```python
from build123d import *

# Parameters (mm, degrees)
SKETCH1_W               = 90
SKETCH1_H               = 52
BOSS_EXTRUDE1_DEPTH     = 3
BOSS_EXTRUDE2_START     = 3
SKETCH4_R               = 2.5
BOSS_EXTRUDE2_DEPTH     = 7
CUT_EXTRUDE2_DEPTH      = 53.92447449
CUT_EXTRUDE2_DEPTH_BACK = 63.92447449
CUT_EXTRUDE2_START      = 10
SKETCH5_R               = 1.35
BOSS_EXTRUDE3_START     = 10
SKETCH6_R               = 0.9
BOSS_EXTRUDE3_DEPTH     = 12.5
SKETCH7_W               = 87
SKETCH7_H               = 49
SKETCH7_W_2             = 81
SKETCH7_H_2             = 43
BOSS_EXTRUDE4_DEPTH     = 2
FILLET1_R               = 3
BOSS_EXTRUDE8_START     = 3
SKETCH8_W               = 89
SKETCH8_H               = 51
SKETCH8_W_2             = 84
SKETCH8_H_2             = 46
BOSS_EXTRUDE8_DEPTH     = 20
FILLET2_R               = 2
CUT_EXTRUDE3_START      = 42
SKETCH9_W               = 14
SKETCH9_H               = 7
CUT_EXTRUDE3_DEPTH      = 15
BOSS_EXTRUDE9_START     = 44.5
BOSS_EXTRUDE9_DEPTH     = 0.2


with BuildPart() as part:
    # Sketch1 → Boss-Extrude1 (new body)
    with BuildSketch(Plane(origin=(0, 0, 0), x_dir=(1, 0, 0), z_dir=(0, 1, 0))):
        Rectangle(SKETCH1_W, SKETCH1_H)
    extrude(amount=BOSS_EXTRUDE1_DEPTH)

    # Sketch4 → Boss-Extrude2 (add)
    with BuildSketch(Plane(origin=(0, 0, 0), x_dir=(1, 0, 0), z_dir=(0, 1, 0)).offset(BOSS_EXTRUDE2_START)):
        with Locations(Location((29, -19.5, 0), (0, 0, 270))):
            Circle(SKETCH4_R)
        with Locations(Location((-37, 18, 0), (0, 0, 270))):
            Circle(SKETCH4_R)
        with Locations(Location((-37, -16.5, 0), (0, 0, 270))):
            Circle(SKETCH4_R)
    extrude(amount=BOSS_EXTRUDE2_DEPTH)

    # Sketch5 → Cut-Extrude2 (cut, two sides: drawn at the far end of the back side and taken through both)
    with BuildSketch(Plane(origin=(0, 0, 0), x_dir=(1, 0, 0), z_dir=(0, 1, 0)).offset(CUT_EXTRUDE2_START - CUT_EXTRUDE2_DEPTH_BACK)):
        with Locations(Location((-37, 18, 0), (0, 0, 270))):
            Circle(SKETCH5_R)
        with Locations(Location((-37, -16.5, 0), (0, 0, 270))):
            Circle(SKETCH5_R)
    extrude(amount=CUT_EXTRUDE2_DEPTH + CUT_EXTRUDE2_DEPTH_BACK, mode=Mode.SUBTRACT)

    # Sketch6 → Boss-Extrude3 (add)
    with BuildSketch(Plane(origin=(0, 0, 0), x_dir=(1, 0, 0), z_dir=(0, 1, 0)).offset(BOSS_EXTRUDE3_START)):
        with Locations(Location((29, -19.5, 0), (0, 0, 270))):
            Circle(SKETCH6_R)
    extrude(amount=BOSS_EXTRUDE3_DEPTH)

    # Sketch7 → Boss-Extrude4 (add)
    with BuildSketch(Plane(origin=(0, 0, 0), x_dir=(1, 0, 0), z_dir=(0, 1, 0))):
        Rectangle(SKETCH7_W, SKETCH7_H)
        Rectangle(SKETCH7_W_2, SKETCH7_H_2, mode=Mode.SUBTRACT)
    extrude(amount=-BOSS_EXTRUDE4_DEPTH)

    # Fillet1
    fillet1_edges = [part.edges().sort_by_distance(p)[0] for p in [
        (43.5, -1, -24.5),
        (43.5, -1, 24.5),
        (-43.5, -1, 24.5),
        (-43.5, -1, -24.5),
    ]]
    fillet(fillet1_edges, radius=FILLET1_R)

    # Sketch8 → Boss-Extrude8 (add)
    with BuildSketch(Plane(origin=(0, 0, 0), x_dir=(1, 0, 0), z_dir=(0, 1, 0)).offset(BOSS_EXTRUDE8_START)):
        Rectangle(SKETCH8_W, SKETCH8_H)
        Rectangle(SKETCH8_W_2, SKETCH8_H_2, mode=Mode.SUBTRACT)
    extrude(amount=BOSS_EXTRUDE8_DEPTH)

    # Fillet2
    fillet2_edges = [part.edges().sort_by_distance(p)[0] for p in [
        (44.5, 13, -25.5),
        (-44.5, 13, -25.5),
        (-44.5, 13, 25.5),
        (44.5, 13, 25.5),
        (-45, 1.5, -26),
        (45, 1.5, -26),
        (45, 1.5, 26),
        (-45, 1.5, 26),
    ]]
    fillet(fillet2_edges, radius=FILLET2_R)

    # Sketch9 → Cut-Extrude3 (cut)
    with BuildSketch(Plane(origin=(0, 0, 0), x_dir=(0, 0, -1), z_dir=(1, 0, 0)).offset(CUT_EXTRUDE3_START)):
        with Locations((11, 6.5)):
            Rectangle(SKETCH9_W, SKETCH9_H)
    extrude(amount=CUT_EXTRUDE3_DEPTH, mode=Mode.SUBTRACT)

    # Sketch10 → Boss-Extrude9 (add)
    with BuildSketch(Plane(origin=(0, 0, 0), x_dir=(0, 0, -1), z_dir=(1, 0, 0)).offset(BOSS_EXTRUDE9_START)):
        Polygon((18, 3), (18, 10), (4, 10), (4, 3), (3, 3), (3, 11), (19, 11), (19, 3), align=None)
    extrude(amount=BOSS_EXTRUDE9_DEPTH)


solid = part.part
```
Verification items for the finished model (mm, model axes). A direction names the side the tool comes from. Coordinates: 2 decimals unless noted, no trailing zeros. Order: outer loops, then holes, each group sorted by start corner. A loop starts at its lowest first (then second) coordinate and runs counter-clockwise, first axis right, second up. Notation, with made-up numbers: (49.25, 18.5) -> (76.25, 18.5) arc R13 ccw to (76.25, 33.5) -> close; hole circle Ø9 at (5, -2.5). An arc over 180 degrees is marked (long way). Answer as CSV lines item,"result". Start each with the question number.
1) Cross-section at A-A, the plane y = 16. Record the boundary of the cut face in (x, z), then the cut area to 3 significant figures.
2) Material ranges on L1, parallel to X at y = 5, z = 16.5; L2, parallel to Z at x = 4.5, y = 21.25; L3, parallel to X at y = 4.5, z = 9, recorded low to high. Write a range as [from, to].
3) Set-up check for faces 1 (the face through (44.7, 10.3, -11)), 2 (the face through (-38.1, 10, -16.9)), 3 (the face through (-43.9, 13.14, -24.93)): record each of +Z, -Z, +X, -X, +Y, -Y from which the full face is reachable in a straight line by a thin tool's end or side.
4) Cross-section at D-D, the plane x = -37. Give the number of separate pieces and of enclosed holes in the cut face, then the cut area to 3 significant figures.
5) Cross-section at C-C, the plane z = 5. Record the boundary of the cut face in (x, y).
6) Gauge pin test, flat ends, axial feed: pin 1 Ø1.6 at (x, y) = (-1, -1.5) entering from -Z; pin 2 Ø2 at (y, z) = (11, 1) entering from +X; pin 3 Ø4 at (x, y) = (-18, 10.5) entering from -Z. Record the tip position at first contact, or that the pin passes through.
7) Release check for a two-part mould opening along X. For faces 4 (the face through (43.93, 13.14, -24.9)), 5 (the face through (-38.32, 4.93, 16.21)), 6 (the face through (-1, -1, 24.5)) record: released by +X, released by -X, zero draft, split by the parting line, or undercut.
8) Cross-section at B-B, the plane x = 29. Record the boundary of the cut face in (y, z).
Conclusion:
1,outline,"(-44.5, -23.5) arc R2 ccw to (-42.5, -25.5) -> (42.5, -25.5) arc R2 ccw to (44.5, -23.5) -> (44.5, 23.5) arc R2 ccw to (42.5, 25.5) -> (-42.5, 25.5) arc R2 ccw to (-44.5, 23.5) -> close; circle Ø1.8 at (29, 19.5); hole (-42, -23) -> (42, -23) -> (42, 23) -> (-42, 23) -> close"
1,area,"674 mm²"
2,L1,"x = [-44.5, -42], [-39.5, -38.35], [-35.65, -34.5], [42, 44.5]"
2,L2,"z = [-25.5, -23], [23, 25.5]"
2,L3,"x = [-44.5, -42], [42, 44.5]"
3,face 1,"+Z, -Z, +X, +Y"
3,face 2,"+Y"
3,face 3,"-Z, -X, +Y"
4,separate pieces,"3"
4,enclosed holes,"0"
4,area,"284 mm²"
5,outline,"(-45, 0) -> (-43.5, 0) -> (-43.5, -2) -> (-40.5, -2) -> (-40.5, 0) -> (40.5, 0) -> (40.5, -2) -> (43.5, -2) -> (43.5, 0) -> (45, 0) -> (45, 3) -> (44.5, 3) -> (44.5, 23) -> (42, 23) -> (42, 3) -> (-42, 3) -> (-42, 23) -> (-44.5, 23) -> (-44.5, 3) -> (-45, 3) -> close"
6,pin 1,"stops at z = -24.5"
6,pin 2,"stops at x = 44.5"
6,pin 3,"stops at z = -25.5"
7,face 4,"released by +X"
7,face 5,"undercut"
7,face 6,"zero draft"
8,outline,"(-2, -24.5) -> (0, -24.5) -> (0, -26) -> (3, -26) -> (3, -25.5) -> (23, -25.5) -> (23, -23) -> (3, -23) -> (3, 17) -> (10, 17) -> (10, 18.6) -> (22.5, 18.6) -> (22.5, 20.4) -> (10, 20.4) -> (10, 22) -> (3, 22) -> (3, 23) -> (23, 23) -> (23, 25.5) -> (3, 25.5) -> (3, 26) -> (0, 26) -> (0, 24.5) -> (-2, 24.5) -> (-2, 21.5) -> (0, 21.5) -> (0, -21.5) -> (-2, -21.5) -> close"
